Can you work these out from the model? Positions are in its coordinate system, mm. A direction names the side the tool comes from. Give positions to 0.01 mm unless a question says otherwise; leave off trailing zeros. Write each loop counter-clockwise with the first axis right and the second up, starting at its lowest first coordinate (ties: lowest second). Pieces come first, ordered by that corner, then holes. Notation, with made-up numbers: (-26.5, 15) - (-1.5, 15) arc R17 ccw to (-1.5, 39) - close; hole circle Ø4 at (7, -12). An arc over 180 degrees is marked (long way). Return JSON: item names as keys, results as strings. Group by question number.
from build123d import *

# Parameters (mm, degrees)
BOSS_EXTRUDE1_DEPTH = 6.35
FILLET1_R           = 10


with BuildPart() as part:
    # Sketch1 → Boss-Extrude1 (new body)
    with BuildSketch(Plane(origin=(0, 0, 0), x_dir=(0, 0, -1), z_dir=(1, 0, 0))):
        with BuildLine():
            Line((-6, 108.391086322), (-6, 16.970562748))
            Line((-6, 16.970562748), (-12, 10.970562748))
            Line((-12, 10.970562748), (-12, -6))
            Line((-12, -6), (12, -6))
            Line((12, -6), (12, 10.970562748))
            Line((12, 10.970562748), (6, 16.970562748))
            Line((6, 16.970562748), (6, 108.391086322))
            ThreePointArc((6, 108.391086322), (11.35412315, 113.306709465), (13.335, 120.3))
            Line((13.335, 120.3), (10.4648, 120.3))
            ThreePointArc((10.4648, 120.3), (0, 130.7648), (-10.4648, 120.3))
            Line((-10.4648, 120.3), (-13.335, 120.3))
            ThreePointArc((-13.335, 120.3), (-11.35412315, 113.306709465), (-6, 108.391086322))
        make_face()
        with BuildLine():
            Line((-3.146426545, 6.425), (3.146426545, 6.425))
            ThreePointArc((3.146426545, 6.425), (0, 2.825), (-3.146426545, 6.425))
        make_face(mode=Mode.SUBTRACT)
    extrude(amount=BOSS_EXTRUDE1_DEPTH)

    # Fillet1
    fillet1_edges = [part.edges().sort_by_distance(p)[0] for p in [
        (3.175, 16.970562748, -6),
        (3.175, 10.970562748, -12),
        (3.175, -6, -12),
        (3.175, -6, 12),
        (3.175, 10.970562748, 12),
        (3.175, 16.970562748, 6),
    ]]
    fillet(fillet1_edges, radius=FILLET1_R)


solid = part.part
1) We'd pull the mould along Y, two halves only. Please class faces 1 (the face through (3, 5, 12)), 2 (the face through (3, 120.3, -12)), 3 (the face through (3.13, 113.22, -11.3)): pulls with the +Y half, pulls with the -Y half, needs draft (parallel to the pull), parting line crosses it, or undercut.
2) Imagine slicing it at C-C, the plane y = 53. Write out the boundary of the cut face in (x, z), and give its area (3 significant figures).
3) I need wall thicknesses on line 1 along Y through (x, z) = (2.25, 0) (3 decimals); line 2 along Z through (x, y) = (2.5, 6) (3 decimals); line 3 along Z through (x, y) = (1.75, 38.5). Which ranges of each line are inside material? Lowest first, please.
4) On a 3-axis mill with a long thin cutter (end or side, diameter ignored), from which of +Z, -Z, +X, -X, +Y, -Y can I reach the whole of each face in a straight line? I mean faces 4 (the face through (3.22, 17.24, -6.78)), 5 (the face through (3, 6.425, 0)), 6 (the face through (3, 5, -12)). Say none if no direction works.
5) Imagine slicing it at A-A, the plane z = 0. Write out the boundary of the cut face in (x, y) (3 decimals), and give its area (3 significant figures).
6) Will these pins go through, and if not, where does the flat tip stop? pin 1 Ø5 at (y, z) = (94, -10.5) entering from +X; pin 2 Ø2.5 at (x, y) = (3.5, 5.5) entering from -Z; pin 3 Ø1 at (x, z) = (4.5, 6.5) entering from -Y; pin 4 Ø0.9 at (x, z) = (3, 11.5) entering from +Y.
Resolved:
{
 "1": {"face 1": "needs draft", "face 2": "pulls with the +Y half", "face 3": "undercut"},
 "2": {"outline": "(0, -6) - (6.35, -6) - (6.35, 6) - (0, 6) - close", "area": "76.2 mm^2"},
 "3": {"line 1": "-6 to 2.825, 6.425 to 130.765", "line 2": "-12 to -3.175, 3.175 to 12", "line 3": "-6 to 6"},
 "4": {"face 4": "-Z, +X, -X", "face 5": "+X, -X", "face 6": "-Z, +X, -X, -Y"},
 "5": {"outline": "(0, -6) - (6.35, -6) - (6.35, 2.825) - (0, 2.825) - close; (0, 6.425) - (6.35, 6.425) - (6.35, 130.765) - (0, 130.765) - close", "area": "846 mm^2"},
 "6": {"pin 1": "through", "pin 2": "z = -12", "pin 3": "y = -5.17", "pin 4": "y = 120.3"}
}
